Work out the finished part from the listing and answer in its coordinate system (mm). Face numbers are marked on the shaded views. A direction names the side the tool comes from. Give positions to 0.01 mm unless a question says otherwise; leave off trailing zeros. Write each loop counter-clockwise with the first axis right and the second up, starting at its lowest first coordinate (ties: lowest second). Pieces come first, ordered by that corner, then holes.
1) Find section A-A (x = 6.5). Determine the outline of the cut face in (y, z), plus the area to 3 significant figures.
2) Find section C-C (z = 0). Count the separate pieces of the cut face and the enclosed holes in it, plus the area to 4 significant figures.
3) Find section B-B (y = 11.7). Determine the outline of the cut face in (x, z), plus the area to 3 significant figures.
4) Straight lines are drawn through the part: probe 1 along X at (y, z) = (0.4, 0); probe 2 along Y at (x, z) = (3, 11.5); probe 3 along X at (y, z) = (22.4, 0). For each, find the intervals that lie inside material, in ascending order.
5) Given pin 1 Ø1 at (x, z) = (-18, -13.5) entering from -Y; pin 2 Ø2 at (x, z) = (-5, -8) entering from +Y; pin 3 Ø2.5 at (x, z) = (-22, 0) entering from +Y, each flat-ended and moving along its own axis, determine where each tip first touches the part or whether it passes through.
6) A tool of negligible diameter and unlimited length cuts with its end or side. For the marked faces 1, 2 and 3, from which of +Z, -Z, +X, -X, +Y, -Y can it reach the whole face along a straight path? Write none if from no direction.
7) Determine the mould class of the marked faces 4, 5 and 6 for opening direction Y: pulls with the +Y half, pulls with the -Y half, needs draft (parallel to the pull), parting line crosses it, or undercut.
```python
from build123d import *

# Parameters (mm, degrees)
SKETCH_12_W          = 64
SKETCH_12_H          = 38.4
EXTRUDE_2_DEPTH      = 23.4
SKETCH_13_W          = 34.4
SKETCH_13_H          = 19.4
CUT_EXTRUDE_10_DEPTH = 71.796892587
SKETCH_14_R          = 4
SKETCH_14_R_2        = 1.1
EXTRUDE_3_DEPTH      = 2
CUT_EXTRUDE_11_DEPTH = 56.191666038
CUT_EXTRUDE_13_REACH = 47.142
SKETCH_17_R          = 1.1
SKETCH_18_R          = 2
CUT_EXTRUDE_14_DEPTH = 1.5
SKETCH_20_W          = 32
SKETCH_20_H          = 32
EXTRUDE_5_DEPTH      = 8.6
SKETCH_21_W          = 28
SKETCH_21_H          = 6.6
CUT_EXTRUDE_16_DEPTH = 61.8
SKETCH_23_W          = 18
SKETCH_23_H          = 22
CUT_EXTRUDE_18_DEPTH = 2
SKETCH_22_R          = 4
CUT_EXTRUDE_17_DEPTH = 30


with BuildPart() as part:
    # 草图12 → 凸台-拉伸2 (new body)
    with BuildSketch(Plane(origin=(0, 0, 0), x_dir=(1, 0, 0), z_dir=(0, 1, 0))):
        Rectangle(SKETCH_12_W, SKETCH_12_H)
    extrude(amount=EXTRUDE_2_DEPTH)

    # 草图13 → 切除-拉伸10 (cut, through all)
    with BuildSketch(Plane(origin=(32, 0, 0), x_dir=(0, 0, -1), z_dir=(1, 0, 0))):
        with Locations((0, 11.7)):
            Rectangle(SKETCH_13_W, SKETCH_13_H)
    extrude(amount=-CUT_EXTRUDE_10_DEPTH, mode=Mode.SUBTRACT)

    # 草图14 → 凸台-拉伸3 (add)
    # profile 1 of 3: a face of its own
    with BuildSketch(Plane.XZ):
        with Locations(Location((-22, 0, 0), (0, 0, 90))):
            Circle(SKETCH_14_R)
        with Locations(Location((-22, 0, 0), (0, 0, 270))):
            Circle(SKETCH_14_R_2, mode=Mode.SUBTRACT)
    # profile 2 of 3: a face of its own
    with BuildSketch(Plane.XZ):
        with Locations(Location((22, 0, 0), (0, 0, 90))):
            Circle(SKETCH_14_R)
        with Locations(Location((22, 0, 0), (0, 0, 90))):
            Circle(SKETCH_14_R_2, mode=Mode.SUBTRACT)
    # profile 3 of 3: a face of its own
    with BuildSketch(Plane.XZ):
        with Locations(Location((0, 0, 0), (0, 0, 90))):
            Circle(SKETCH_14_R)
        with Locations(Location((0, 0, 0), (0, 0, 270))):
            Circle(SKETCH_14_R_2, mode=Mode.SUBTRACT)
    extrude(amount=EXTRUDE_3_DEPTH)

    # 草图15 → 切除-拉伸11 (cut, through all)
    with BuildSketch(Plane.XY.offset(19.2)):
        with BuildLine():
            Line((-20, 19.7), (20, 19.7))
            ThreePointArc((20, 19.7), (28, 11.7), (20, 3.7))
            Line((20, 3.7), (-20, 3.7))
            ThreePointArc((-20, 3.7), (-28, 11.7), (-20, 19.7))
        make_face()
    extrude(amount=-CUT_EXTRUDE_11_DEPTH, mode=Mode.SUBTRACT)

    # 草图17 → 切除-拉伸13 (cut, up to next)
    with BuildSketch(Plane.XZ.offset(2), mode=Mode.PRIVATE) as cut_extrude_13_sk1:
        with Locations(Location((22, 0, 0), (0, 0, 90))):
            Circle(SKETCH_17_R)
    cut_extrude_13_tool1 = extrude(cut_extrude_13_sk1.sketch, amount=-CUT_EXTRUDE_13_REACH, mode=Mode.PRIVATE) & part.part
    # 草图17 → 切除-拉伸13 (cut, up to next)
    with BuildSketch(Plane.XZ.offset(2), mode=Mode.PRIVATE) as cut_extrude_13_sk2:
        with Locations(Location((-22, 0, 0), (0, 0, 270))):
            Circle(SKETCH_17_R)
    cut_extrude_13_tool2 = extrude(cut_extrude_13_sk2.sketch, amount=-CUT_EXTRUDE_13_REACH, mode=Mode.PRIVATE) & part.part
    # 草图17 → 切除-拉伸13 (cut, up to next)
    with BuildSketch(Plane.XZ.offset(2), mode=Mode.PRIVATE) as cut_extrude_13_sk3:
        with Locations(Location((0, 0, 0), (0, 0, 270))):
            Circle(SKETCH_17_R)
    cut_extrude_13_tool3 = extrude(cut_extrude_13_sk3.sketch, amount=-CUT_EXTRUDE_13_REACH, mode=Mode.PRIVATE) & part.part
    add(cut_extrude_13_tool1.solids().sort_by_distance((22, -2, 0))[0], mode=Mode.SUBTRACT)
    add(cut_extrude_13_tool2.solids().sort_by_distance((-22, -2, 0))[0], mode=Mode.SUBTRACT)
    add(cut_extrude_13_tool3.solids().sort_by_distance((0, -2, 0))[0], mode=Mode.SUBTRACT)

    # 草图18 → 切除-拉伸14 (cut)
    with BuildSketch(Plane(origin=(0, 2, 0), x_dir=(1, 0, 0), z_dir=(0, 1, 0))):
        with Locations(Location((-22, 0, 0), (0, 0, 270))):
            Circle(SKETCH_18_R)
        with Locations(Location((22, 0, 0), (0, 0, 270))):
            Circle(SKETCH_18_R)
        with Locations(Location((0, 0, 0), (0, 0, 270))):
            Circle(SKETCH_18_R)
    extrude(amount=-CUT_EXTRUDE_14_DEPTH, mode=Mode.SUBTRACT)

    # 草图20 → 凸台-拉伸5 (add)
    with BuildSketch(Plane(origin=(0, 23.4, 0), x_dir=(1, 0, 0), z_dir=(0, 1, 0))):
        Rectangle(SKETCH_20_W, SKETCH_20_H)
    extrude(amount=EXTRUDE_5_DEPTH)

    # 草图21 → 切除-拉伸16 (cut, through all)
    with BuildSketch(Plane(origin=(16, 0, 0), x_dir=(0, 0, -1), z_dir=(1, 0, 0))):
        with Locations((0, 26.7)):
            Rectangle(SKETCH_21_W, SKETCH_21_H)
    extrude(amount=-CUT_EXTRUDE_16_DEPTH, mode=Mode.SUBTRACT)

    # 草图23 → 切除-拉伸18 (cut)
    with BuildSketch(Plane(origin=(0, 32, 0), x_dir=(1, 0, 0), z_dir=(0, 1, 0))):
        with BuildLine():
            Line((-16, 16), (-16, -16))
            add(Edge.make_bspline(
                [(-16, 16), (-10, 0), (-16, -16)],
                knots=[0, 0, 0, 1, 1, 1], degree=2))
        make_face()
        with BuildLine():
            Line((16, 16), (16, -16))
            add(Edge.make_bspline(
                [(16, 16), (10, 0), (16, -16)],
                knots=[0, 0, 0, 1, 1, 1], degree=2))
        make_face()
        Rectangle(SKETCH_23_W, SKETCH_23_H)
    extrude(amount=-CUT_EXTRUDE_18_DEPTH, mode=Mode.SUBTRACT)

    # 草图22 → 切除-拉伸17 (cut)
    with BuildSketch(Plane(origin=(0, 32, 0), x_dir=(1, 0, 0), z_dir=(0, 1, 0))):
        with Locations(Location((22, 0, 0), (0, 0, 270))):
            Circle(SKETCH_22_R)
        with Locations(Location((-22, 0, 0), (0, 0, 270))):
            Circle(SKETCH_22_R)
        with Locations(Location((0, 0, 0), (0, 0, 270))):
            Circle(SKETCH_22_R)
    extrude(amount=-CUT_EXTRUDE_17_DEPTH, mode=Mode.SUBTRACT)


solid = part.part
```
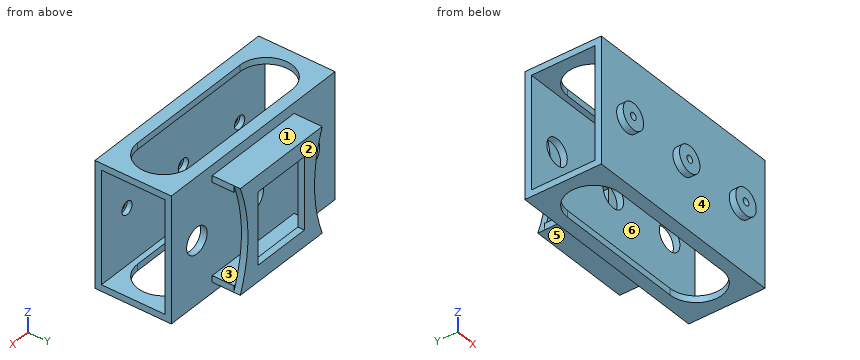
Results:
1. outline: (0, -19.2) - (3.7, -19.2) - (3.7, -17.2) - (2, -17.2) - (2, 17.2) - (3.7, 17.2) - (3.7, 19.2) - (0, 19.2) - close; (19.7, -19.2) - (23.4, -19.2) - (23.4, -16) - (32, -16) - (32, -11) - (30, -11) - (30, -14) - (23.4, -14) - (23.4, 14) - (30, 14) - (30, 11) - (32, 11) - (32, 16) - (23.4, 16) - (23.4, 19.2) - (19.7, 19.2) - (19.7, 17.2) - (21.4, 17.2) - (21.4, -17.2) - (19.7, -17.2) - close
1. area: 214 mm2
2. separate pieces: 10
2. enclosed holes: 0
2. area: 237.5 mm2
3. outline: (-32, -19.2) - (-28, -19.2) - (-28, -17.2) - (-32, -17.2) - close; (-32, 17.2) - (-28, 17.2) - (-28, 19.2) - (-32, 19.2) - close; (28, -19.2) - (32, -19.2) - (32, -17.2) - (28, -17.2) - close; (28, 17.2) - (32, 17.2) - (32, 19.2) - (28, 19.2) - close
3. area: 32.0 mm2
4. probe 1: x = -32 to -23.1, -20.9 to -1.1, 1.1 to 20.9, 23.1 to 32
4. probe 2: y = 0 to 2, 21.4 to 23.4, 30 to 32
4. probe 3: x = -32 to -26, -18 to -4, 4 to 18, 26 to 32
5. pin 1: stops at y = 0
5. pin 2: stops at y = 23.4
5. pin 3: stops at y = 0.5
6. face 1: +Z, +X, -X, +Y
6. face 2: +Z, -Z, +X, -X, +Y
6. face 3: +X, -X
7. face 4: pulls with the -Y half
7. face 5: needs draft
7. face 6: undercut
